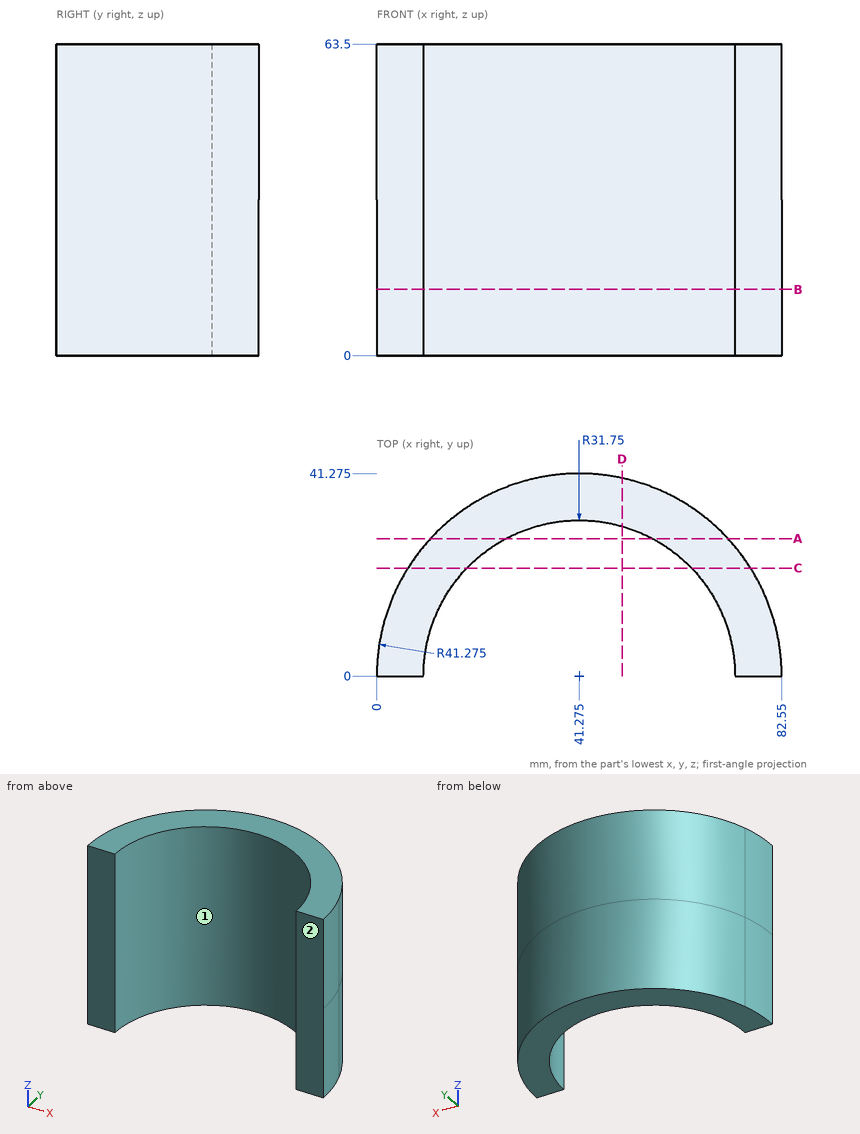
Check sheet for the drawn part. Datum: minimum x, y, z corner. Units: mm. Coordinates: 2 decimals unless noted, no trailing zeros. Loops run counter-clockwise (first coordinate to the right, second up) from the corner with the lowest first, then second, coordinate; pieces in that order, holes last. Notation, with made-up numbers: (0, 53.5) -> (55, 53.5) arc R18 ccw to (55, 73.5) -> close; hole circle Ø3 at (77, 63). An arc over 180 degrees is marked (long way). Answer as a JSON object with one key per item and string values. Group by question number.
Item 1: Sectioned sample at A-A on y = 28. Record the boundary of the cut face in (x, z), plus the area to 3 significant figures.
Item 2: Scan lines: probe 1 along X at (y, z) = (9, 30); probe 2 along X at (y, z) = (29.5, 5); probe 3 along Y at (x, z) = (40.5, 7). Record each from-to range of solid material in increasing order.
Item 3: Depth check by flat-ended pin: pin 1 (2 mm diameter, centred on y = 10, z = 17, fed in from +X); pin 2 (3 mm diameter, centred on y = 22, z = 41, fed in from +X); pin 3 (3 mm diameter, centred on x = 59.5, z = 23.5, fed in from +Y). Enter the tip coordinate at first touch or a pass-through.
Item 4: Sectioned sample at D-D on x = 50. Record the boundary of the cut face in (y, z), plus the area to 3 significant figures.
Item 5: Mould release check, pull along X, two halves, no side actions. Record for the marked faces 1 and 2: +X half, -X half, draft (parallel to the pull), parting line (faces both ways), or undercut.
Item 6: Sectioned sample at B-B on z = 13.5. Record the boundary of the cut face in (x, y) (3 decimals).
Item 7: Sectioned sample at C-C on y = 22. Record the boundary of the cut face in (x, z).
Evaluation:
{
 "1": {"outline": "(10.95, 0) -> (26.31, 0) -> (26.31, 63.5) -> (10.95, 63.5) -> close; (56.24, 0) -> (71.6, 0) -> (71.6, 63.5) -> (56.24, 63.5) -> close", "area": "1,950 mm²"},
 "2": {"probe 1": "x = 0.99 to 10.83, 71.72 to 81.56", "probe 2": "x = 12.41 to 29.54, 53.01 to 70.14", "probe 3": "y = 31.74 to 41.27"},
 "3": {"pin 1": "stops at x = 81.56", "pin 2": "stops at x = 77.1", "pin 3": "stops at y = 37.73"},
 "4": {"outline": "(30.53, 0) -> (40.34, 0) -> (40.34, 63.5) -> (30.53, 63.5) -> close", "area": "623 mm²"},
 "5": {"face 1": "undercut", "face 2": "draft"},
 "6": {"outline": "(0, 0) -> (9.525, 0) arc R31.75 cw to (73.025, 0) -> (82.55, 0) arc R41.275 ccw to start"},
 "7": {"outline": "(6.35, 0) -> (18.38, 0) -> (18.38, 63.5) -> (6.35, 63.5) -> close; (64.17, 0) -> (76.2, 0) -> (76.2, 63.5) -> (64.17, 63.5) -> close"}
}
